from build123d import *

# Parameters (mm, degrees)
BOSS_EXTRU_1_DEPTH      = 12.7
ESQUISSE2_R             = 3.175
ENL_V_MAT_EXTRU_1_DEPTH = 120.412691269
ENL_V_MAT_EXTRU_2_DEPTH = 120.412691269


with BuildPart() as part:
    # Esquisse1 → Boss.-Extru.1 (new body)
    with BuildSketch(Plane.XY):
        with BuildLine():
            Line((34.925, -85.344), (34.925, -71.788707818))
            ThreePointArc((34.925, -71.788707818), (41.275, -24.644), (47.625, -71.788707818))
            Line((47.625, -71.788707818), (47.625, -85.344))
            Line((47.625, -85.344), (82.55, -85.344))
            Line((82.55, -85.344), (82.55, 0))
            Line((82.55, 0), (0, 0))
            Line((0, 0), (0, -85.344))
            Line((0, -85.344), (34.925, -85.344))
        make_face()
    extrude(amount=BOSS_EXTRU_1_DEPTH)

    # Esquisse2 → Enlèv. mat.-Extru.1 (cut, through all)
    with BuildSketch(Plane(origin=(82.55, 0, 0), x_dir=(0, 0, -1), z_dir=(1, 0, 0))):
        with Locations(Location((-6.35, -78.994, 0), (0, 0, 90))):
            Circle(ESQUISSE2_R)
    extrude(amount=-ENL_V_MAT_EXTRU_1_DEPTH, mode=Mode.SUBTRACT)

    # Esquisse4 → Enlèvement de matière-Révolution1 (revolve, cut)
    with BuildSketch(Plane.XZ.offset(48.644)):
        Polygon((17.275, 12.7), (14.533802376, -0.19632088), (34.925, -0.19632088), (34.925, 12.7), align=None)
    revolve(axis=Axis((41.275, -48.644, 0), (0, 0, 1)), mode=Mode.SUBTRACT)

    # Esquisse5 → Enlèv. mat.-Extru.2 (cut, through all)
    with BuildSketch(Plane(origin=(0, 0, 0), x_dir=(-1, 0, 0), z_dir=(0, 0, -1))):
        Polygon((-71.501, 0), (-82.55, -21.684883475), (-82.55, 0), align=None)
        Polygon((-11.049, 0), (0, -21.684883475), (0, 0), align=None)
    extrude(amount=-ENL_V_MAT_EXTRU_2_DEPTH, mode=Mode.SUBTRACT)


solid = part.part
Could you check a few things on this model? Use its own coordinates, in mm. A direction names the side the tool comes from. Round coordinates to 2 decimals unless told otherwise and drop trailing zeros. Loops run counter-clockwise (first coordinate to the right, second up) from the corner with the lowest first, then second, coordinate; pieces in that order, holes last. Notation, with made-up numbers: (23, 6.5) -> (82, 6.5) arc R15 cw to (82, 34.5) -> close; hole circle Ø7 at (3, 34). An arc over 180 degrees is marked (long way). Use CSV: the item, a comma, the result in double quotes.
(1) For faces 4 (the flat face through (34.925, -75.6, 6.3)), 5 (the flat face through (17, -85.344, 6)), which set-ups out of +Z, -Z, +X, -X, +Y, -Y let a thin tool reach every point of the face, with its end or its side?
Return value:
face 4,"+Z, -Z, -Y"
face 5,"+Z, -Z, +X, -X, -Y"
(2) Will this pin go through, and if not, where does the flat tip stop? pin 1 Ø5 at (y, z) = (-78.994, 6.35) entering from -X.
Return value:
pin 1,"passes through"
(3) If I drill on probe 1 along X at (y, z) = (-75, 6.25) (3 decimals); probe 2 along Y at (x, z) = (11.5, 5.25); probe 3 along Y at (x, z) = (13.5, 4.5), over which ranges is the centre line in solid material (lowest first)? Write a range as [from, to].
Return value:
probe 1,"x = [0, 34.925], [47.625, 82.55]"
probe 2,"y = [-85.34, -81.97], [-76.02, 0]"
probe 3,"y = [-85.34, -81.57], [-76.41, 0]"
(4) Suppose I cut it at C-C on z = 10.75. Write out the boundary of the cut face in (x, y) (3 decimals).
Return value:
outline,"(0, -85.344) -> (34.925, -85.344) -> (34.925, -72.218) arc R24.414 cw (long way) to (47.625, -72.218) -> (47.625, -85.344) -> (82.55, -85.344) -> (82.55, -21.685) -> (71.501, 0) -> (11.049, 0) -> (0, -21.685) -> close"
(5) Suppose I cut it at A-A on z = 6.35. Write out the boundary of the cut face in (x, y) (3 decimals).
Return value:
outline,"(0, -85.344) -> (34.925, -85.344) -> (34.925, -82.169) -> (0, -82.169) -> close; (0, -75.819) -> (34.925, -75.819) -> (34.925, -73.186) arc R25.35 cw (long way) to (47.625, -73.186) -> (47.625, -75.819) -> (82.55, -75.819) -> (82.55, -21.685) -> (71.501, 0) -> (11.049, 0) -> (0, -21.685) -> close; (47.625, -85.344) -> (82.55, -85.344) -> (82.55, -82.169) -> (47.625, -82.169) -> close"
(6) If we mould it in two halves opening along X, with no side actions, what happens to faces 1 (the flat face through (82.55, -54, 6)), 2 (the flat face through (47.625, -77, 9.1)), 3 (the flat face through (50, -23, 0))? For each: +X half, -X half, draft (parallel to the pull), parting line (faces both ways), or undercut.
Return value:
face 1,"+X half"
face 2,"undercut"
face 3,"draft"
(7) Suppose I cut it at D-D on x = 28. Give the number of separate pieces and of enclosed holes in the cut face, plus the area to 3 significant figures.
Return value:
separate pieces,"2"
enclosed holes,"1"
area,"504 mm²"
(8) Suppose I cut it at B-B on x = 73.5. Write out the boundary of the cut face in (y, z) (3 decimals), plus the area to 3 significant figures.
Return value:
outline,"(-85.344, 0) -> (-3.923, 0) -> (-3.923, 12.7) -> (-85.344, 12.7) -> close; hole circle Ø6.35 at (-78.994, 6.35)"
area,"1,000 mm²"
